```python
from build123d import *

# Parameters (mm, degrees)
SKETCH_1_R               = 110
EXTRUDE_1_DEPTH          = 3
CUT_EXTRUDE_1_DEPTH      = 156.592416268
CUT_EXTRUDE_1_DEPTH_BACK = 156.592416268
SKETCH_2_R               = 2.05
SKETCH_4_R               = 5
CUT_EXTRUDE_2_DEPTH      = 1.5


with BuildPart() as part:
    # 草图1 → 凸台-拉伸1 (new body)
    with BuildSketch(Plane(origin=(0, 0, 0), x_dir=(1, 0, 0), z_dir=(0, 1, 0))):
        with Locations(Location((0, 0, 0), (0, 0, 270))):
            Circle(SKETCH_1_R)
    extrude(amount=EXTRUDE_1_DEPTH)

    # 草图2 → 切除-拉伸1 (cut, two sides: drawn at the far end of the back side and taken through both)
    with BuildSketch(Plane(origin=(0, 3, 0), x_dir=(1, 0, 0), z_dir=(0, 1, 0)).offset(-CUT_EXTRUDE_1_DEPTH_BACK)):
        with Locations(Location((20, 22, 0), (0, 0, 270))):
            Circle(SKETCH_2_R)
        with Locations(Location((0, 22, 0), (0, 0, 270))):
            Circle(SKETCH_2_R)
        with Locations(Location((0, 42, 0), (0, 0, 270))):
            Circle(SKETCH_2_R)
        with Locations(Location((0, 2, 0), (0, 0, 270))):
            Circle(SKETCH_2_R)
        with Locations(Location((-20, 22, 0), (0, 0, 270))):
            Circle(SKETCH_2_R)
    extrude(amount=CUT_EXTRUDE_1_DEPTH + CUT_EXTRUDE_1_DEPTH_BACK, mode=Mode.SUBTRACT)

    # 草图4 → 切除-拉伸2 (cut)
    with BuildSketch(Plane(origin=(0, 3, 0), x_dir=(1, 0, 0), z_dir=(0, 1, 0))):
        with Locations(Location((0, 22, 0), (0, 0, 270))):
            Circle(SKETCH_4_R)
        with Locations(Location((20, 22, 0), (0, 0, 270))):
            Circle(SKETCH_4_R)
        with Locations(Location((0, 42, 0), (0, 0, 270))):
            Circle(SKETCH_4_R)
        with Locations(Location((0, 2, 0), (0, 0, 270))):
            Circle(SKETCH_4_R)
        with Locations(Location((-20, 22, 0), (0, 0, 270))):
            Circle(SKETCH_4_R)
    extrude(amount=-CUT_EXTRUDE_2_DEPTH, mode=Mode.SUBTRACT)


solid = part.part
```
Part model, mm, in its own coordinate system. A direction names the side the tool comes from. Coordinates: 2 decimals unless noted, no trailing zeros. Write each loop counter-clockwise with the first axis right and the second up, starting at its lowest first coordinate (ties: lowest second). Pieces come first, ordered by that corner, then holes.
Item 1: Slice it at A-A (y = 2.05). Write the cut outline in (x, z), and give its area (3 significant figures).
Item 2: Slice it at C-C (x = 38). Write the cut outline in (y, z).
Item 3: Slice it at B-B (z = 34). Write the cut outline in (x, y).
Item 4: Pin check, flat tips, straight feed: pin 1 (13 mm diameter, centred on x = 0, z = -22, fed in from -Y); pin 2 (1 mm diameter, centred on y = 1.5, z = 38.5, fed in from +X); pin 3 (1.5 mm diameter, centred on x = 28, y = 1.5, fed in from -Z); pin 4 (3.5 mm diameter, centred on x = 0, z = -42, fed in from -Y). Stop position of each tip, or through.
Item 5: Probe line 1 (X direction, y = 0.5, z = 1); line 2 (X direction, y = 2.25, z = -22); line 3 (Z direction, x = 20, y = 0.8). List the from-to ranges inside material, lowest first.
Item 6: Which spindle directions (+Z, -Z, +X, -X, +Y, -Y) get a long thin tool onto all of the face, cutting with end or side? Do faces 1 (the face through (0.1, 1.5, -39.8)), 2 (the face through (2, 3, 23)). Say none if no direction does.
Item 7: Mould opens along Z. For faces 3 (the face through (-23, 0, -2)), 4 (the face through (-97.59, 1.48, 50.76)), 5 (the face through (0, 2, -27)) say: released by +Z, released by -Z, zero draft, split by the parting line, or undercut.
Results found:
1. outline: circle Ø220 at (0, 0); hole circle Ø10 at (-20, -22); hole circle Ø10 at (0, -42); hole circle Ø10 at (0, -22); hole circle Ø10 at (0, -2); hole circle Ø10 at (20, -22)
1. area: 37,600 mm2
2. outline: (0, -103.23) - (3, -103.23) - (3, 103.23) - (0, 103.23) - close
3. outline: (-104.61, 0) - (104.61, 0) - (104.61, 3) - (-104.61, 3) - close
4. pin 1: stops at y = 0
4. pin 2: stops at x = 103.23
4. pin 3: stops at z = -106.57
4. pin 4: passes through
5. line 1: x = -110 to 110
5. line 2: x = -107.78 to -25, -15 to -5, 5 to 15, 25 to 107.78
5. line 3: z = -108.17 to -24.05, -19.95 to 108.17
6. face 1: +Y
6. face 2: +Z, -Z, +X, -X, +Y
7. face 3: zero draft
7. face 4: split by the parting line
7. face 5: undercut
